Read the model definition and answer for the solid it produces. Units are mm, in the model's axes. Give positions to 0.01 mm unless a question says otherwise; leave off trailing zeros. Order: outer loops, then holes, each group sorted by start corner. A loop starts at its lowest first (then second) coordinate and runs counter-clockwise, first axis right, second up. Notation, with made-up numbers: (-10.75, 74) - (-3.75, 74) arc R26 cw to (-3.75, 109) - close; hole circle Ø7 at (-1, 59). An arc over 180 degrees is marked (long way). Answer as CSV lines item,"result". Start each with the question number.
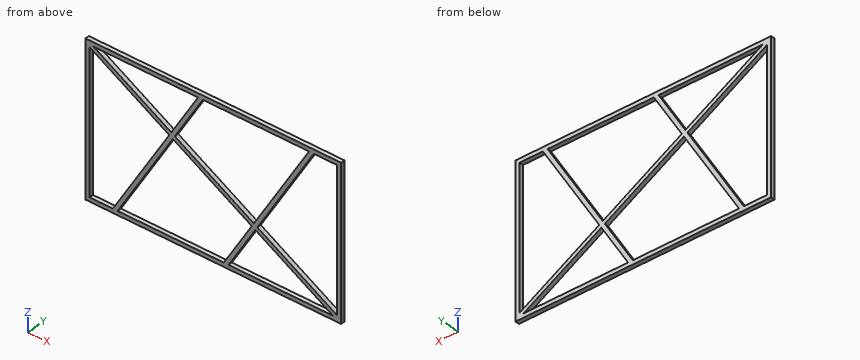
from build123d import *

# Parameters (mm, degrees)
F0_W     = 2500
F0_H     = 1500
F1_DEPTH = 40


with BuildPart() as f1:
    # F0 (on Front) → F1 (new body)
    with BuildSketch(Plane.XZ):
        with Locations((1250, 750)):
            Rectangle(F0_W, F0_H)
        Polygon((40, 1436.8111485162), (40, 1460), (79.5190285851, 1460), (1100.8899553859, 1460), (1147.2676583536, 1460), (2185.9554821423, 1460), (2232.33318511, 1460), (2460, 1460), (2460, 63.1888514838), (2460, 40), (2420.4809714149, 40), (1399.1100446141, 40), (1352.7323416464, 40), (314.0445178577, 40), (267.66681489, 40), (40, 40), align=None, mode=Mode.SUBTRACT)
        Polygon((853.5499625474, 959.4388564429), (819.0506256329, 979.6822690125), (267.66681489, 40), (314.0445178577, 40), align=None)
        Polygon((79.5190285851, 1460), (40, 1460), (40, 1436.8111485162), (819.0506256329, 979.6822690125), (839.2940382026, 1014.181605927), align=None)
        Polygon((873.793375117, 993.9381933573), (839.2940382026, 1014.181605927), (819.0506256329, 979.6822690125), (853.5499625474, 959.4388564429), align=None)
        Polygon((1147.2676583536, 1460), (1100.8899553859, 1460), (839.2940382026, 1014.181605927), (873.793375117, 993.9381933573), align=None)
        Polygon((1646.4500374526, 540.5611435571), (873.793375117, 993.9381933573), (853.5499625474, 959.4388564429), (1626.206624883, 506.0618066427), align=None)
        Polygon((2232.33318511, 1460), (2185.9554821423, 1460), (1646.4500374526, 540.5611435571), (1680.9493743671, 520.3177309875), align=None)
        Polygon((2460, 63.1888514838), (1680.9493743671, 520.3177309875), (1660.7059617974, 485.818394073), (2420.4809714149, 40), (2460, 40), align=None)
        Polygon((1680.9493743671, 520.3177309875), (1646.4500374526, 540.5611435571), (1626.206624883, 506.0618066427), (1660.7059617974, 485.818394073), align=None)
        Polygon((1660.7059617974, 485.818394073), (1626.206624883, 506.0618066427), (1352.7323416464, 40), (1399.1100446141, 40), align=None)
    extrude(amount=F1_DEPTH)


solid = f1.part
(1) A flat-ended cylindrical pin translates along its axis: pin 1 Ø1 at (x, z) = (1484.5, 637) entering from +Y. Find the tip coordinate at first contact, or state that the pin passes through.
(2) Section B-B, the plane z = 1060.5 is taken. Write down the section's boundary in (x, y), and give its area (3 significant figures).
(3) Straight lines are drawn through the part: line 1 (Z direction, x = 1196.5, y = -29); line 2 (Z direction, x = 2220, y = -19); line 3 (X direction, y = -18.5, z = 386). For each, find the intervals that lie inside material, in ascending order. Write a range as [from, to].
(4) Section C-C, the plane x = 1329 is taken. Write down the section's boundary in (y, z).
(5) Section A-A, the plane y = -29 is taken. Write down the section's boundary in (x, z), and give its area (3 significant figures).
Checks:
1,pin 1,"passes through"
2,outline,"(0, -40) - (40, -40) - (40, 0) - (0, 0) - close; (681.32, -40) - (760.36, -40) - (760.36, 0) - (681.32, 0) - close; (866.47, -40) - (912.85, -40) - (912.85, 0) - (866.47, 0) - close; (1951.54, -40) - (1997.92, -40) - (1997.92, 0) - (1951.54, 0) - close; (2460, -40) - (2500, -40) - (2500, 0) - (2460, 0) - close"
2,area,"10,100 mm²"
3,line 1,"z = [0, 40], [758.2, 804.58], [1460, 1500]"
3,line 2,"z = [0, 40], [157.64, 204.02], [1438.98, 1500]"
3,line 3,"x = [0, 40], [470.69, 517.07], [1555.76, 1602.13], [1830.82, 1909.86], [2460, 2500]"
4,outline,"(-40, 0) - (0, 0) - (0, 40) - (-40, 40) - close; (-40, 680.46) - (0, 680.46) - (0, 726.83) - (-40, 726.83) - close; (-40, 1460) - (0, 1460) - (0, 1500) - (-40, 1500) - close"
5,outline,"(0, 0) - (2500, 0) - (2500, 1500) - (0, 1500) - close; hole (40, 40) - (267.67, 40) - (819.05, 979.68) - (40, 1436.81) - close; hole (79.52, 1460) - (839.29, 1014.18) - (1100.89, 1460) - close; hole (314.04, 40) - (1352.73, 40) - (1626.21, 506.06) - (853.55, 959.44) - close; hole (873.79, 993.94) - (1646.45, 540.56) - (2185.96, 1460) - (1147.27, 1460) - close; hole (1399.11, 40) - (2420.48, 40) - (1660.71, 485.82) - close; hole (1680.95, 520.32) - (2460, 63.19) - (2460, 1460) - (2232.33, 1460) - close"
5,area,"553,000 mm²"
